Build history of the part. All positions in model axes, mm. Face numbers are marked on the shaded views. A direction names the side the tool comes from. Coordinates: 2 decimals unless noted, no trailing zeros. Write each loop counter-clockwise with the first axis right and the second up, starting at its lowest first coordinate (ties: lowest second). Pieces come first, ordered by that corner, then holes. Notation, with made-up numbers: (22, 68) -> (59, 68) arc R20 ccw to (59, 80) -> close; hole circle Ø5 at (-14.5, 89.5). An arc over 180 degrees is marked (long way). Write each question's results on one line, items separated by ' | '. Start each with the question number.
Q1. Drill centre lines: line 1 (Y direction, x = -17, z = -4.5); line 2 (Y direction, x = 2.5, z = -16.5); line 3 (X direction, y = 3.5, z = -12). Where is each one in solid material? Low to high.
Q2. Saw through at B-B on x = -17. Give the cut face in (y, z), and give its area (3 significant figures).
Q3. Saw through at C-C on z = -5. Give the cut face in (x, y), and give its area (3 significant figures).
Q4. Drop flat-ended pins along their axis: pin 1 Ø3.5 at (y, z) = (26.5, -26) entering from -X; pin 2 Ø9 at (x, y) = (17, 15) entering from +Z; pin 3 Ø1 at (x, y) = (-0.5, 14) entering from +Z; pin 4 Ø10 at (y, z) = (9, -25.5) entering from +X. Give the stop position or say it passes through.
Q5. Two-plate mould, pull along Z, no slides. Class the marked faces 1, 2, 3 and 4: released by +Z, released by -Z, zero draft, split by the parting line, or undercut.
Q6. Tool access for the marked faces 5, 6 and 7: list every direction of +Z, -Z, +X, -X, +Y, -Y with a clear straight run to the whole face (end or side of a thin tool).
Q7. Saw through at A-A on y = 15. Count the separate pieces of the cut face and the enclosed holes in it, and give its area (3 significant figures).
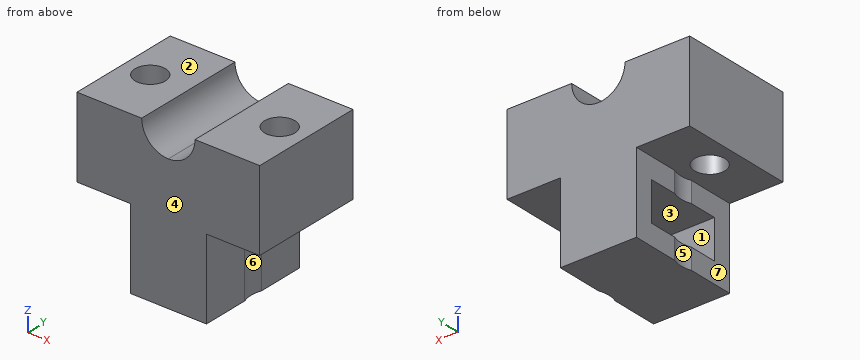
from build123d import *

# Parameters (mm, degrees)
SKETCH_1_W          = 48
SKETCH_1_H          = 20
EXTRUDE_1_DEPTH     = 30
SKETCH_2_W          = 14
SKETCH_2_H          = 30
CUT_EXTRUDE_1_DEPTH = 7
SKETCH_7_W          = 22
SKETCH_7_H          = 30
EXTRUDE_2_DEPTH     = 48
SKETCH_8_W          = 21
SKETCH_8_H          = 30
CUT_EXTRUDE_2_DEPTH = 14
SKETCH_9_W          = 21
SKETCH_9_H          = 30
CUT_EXTRUDE_3_DEPTH = 14
SKETCH_11_W         = 10.2
SKETCH_11_H         = 20.2
CUT_EXTRUDE_4_DEPTH = 56.497747702
SKETCH_13_R         = 4
CUT_EXTRUDE_5_DEPTH = 44.783558558
SKETCH_14_R         = 4
CUT_EXTRUDE_6_DEPTH = 44.783558558
FILLET_1_R          = 7
SKETCH1_W           = 10.2
SKETCH1_H           = 20.2
BOSS_EXTRUDE1_DEPTH = 4
SKETCH_20_R         = 7.5
CUT_EXTRUDE_8_DEPTH = 44.783558558


with BuildPart() as part:
    # Эскиз1 → Бобышка-Вытянуть1 (new body)
    with BuildSketch(Plane(origin=(0, 0, 0), x_dir=(1, 0, 0), z_dir=(0, 1, 0))):
        Rectangle(SKETCH_1_W, SKETCH_1_H)
    extrude(amount=EXTRUDE_1_DEPTH)

    # Эскиз2 → Вырез-Вытянуть1 (cut)
    with BuildSketch(Plane.XY.offset(10)):
        with Locations((0, 15)):
            Rectangle(SKETCH_2_W, SKETCH_2_H)
    extrude(amount=-CUT_EXTRUDE_1_DEPTH, mode=Mode.SUBTRACT)

    # Эскиз7 → Бобышка-Вытянуть2 (add)
    with BuildSketch(Plane(origin=(24, 0, 0), x_dir=(0, 0, -1), z_dir=(1, 0, 0))):
        with Locations((21, 15)):
            Rectangle(SKETCH_7_W, SKETCH_7_H)
    extrude(amount=-EXTRUDE_2_DEPTH)

    # Эскиз8 → Вырез-Вытянуть2 (cut)
    with BuildSketch(Plane(origin=(24, 0, 0), x_dir=(0, 0, -1), z_dir=(1, 0, 0))):
        with Locations((21.5, 15)):
            Rectangle(SKETCH_8_W, SKETCH_8_H)
    extrude(amount=-CUT_EXTRUDE_2_DEPTH, mode=Mode.SUBTRACT)

    # Эскиз9 → Вырез-Вытянуть3 (cut)
    with BuildSketch(Plane.ZY.offset(24)):
        with Locations((-21.5, 15)):
            Rectangle(SKETCH_9_W, SKETCH_9_H)
    extrude(amount=-CUT_EXTRUDE_3_DEPTH, mode=Mode.SUBTRACT)

    # Эскиз11 → Вырез-Вытянуть4 (cut, through all)
    with BuildSketch(Plane.ZY.offset(10)):
        with Locations((-21.5, 15)):
            Rectangle(SKETCH_11_W, SKETCH_11_H)
    extrude(amount=-CUT_EXTRUDE_4_DEPTH, mode=Mode.SUBTRACT)

    # Эскиз13 → Вырез-Вытянуть5 (cut, through all)
    with BuildSketch(Plane(origin=(0, 0, -11), x_dir=(-1, 0, 0), z_dir=(0, 0, -1))):
        with Locations((17, 15)):
            Circle(SKETCH_13_R)
    extrude(amount=-CUT_EXTRUDE_5_DEPTH, mode=Mode.SUBTRACT)

    # Эскиз14 → Вырез-Вытянуть6 (cut, through all)
    with BuildSketch(Plane(origin=(0, 0, -11), x_dir=(-1, 0, 0), z_dir=(0, 0, -1))):
        with Locations((-17, 15)):
            Circle(SKETCH_14_R)
    extrude(amount=-CUT_EXTRUDE_6_DEPTH, mode=Mode.SUBTRACT)

    # Скругление1
    fillet_1_edges = [part.edges().sort_by_distance(p)[0] for p in [
        (-7, 15, 3),
        (7, 15, 3),
    ]]
    fillet(fillet_1_edges, radius=FILLET_1_R - 0.0001)  # a hair under: the kernel refuses the full size

    # Sketch1 → Boss-Extrude1 (add)
    with BuildSketch(Plane(origin=(10, 0, 0), x_dir=(0, 0, -1), z_dir=(1, 0, 0))):
        with Locations((21.5, 15)):
            Rectangle(SKETCH1_W, SKETCH1_H)
    extrude(amount=-BOSS_EXTRUDE1_DEPTH)

    # Эскиз20 → Вырез-Вытянуть8 (cut, through all)
    with BuildSketch(Plane(origin=(0, 0, -11), x_dir=(-1, 0, 0), z_dir=(0, 0, -1))):
        with Locations((-17, 15)):
            Circle(SKETCH_20_R)
        with Locations((17, 15)):
            Circle(SKETCH_20_R)
    extrude(amount=CUT_EXTRUDE_8_DEPTH, mode=Mode.SUBTRACT)


solid = part.part
Returned:
1) line 1: y = 0 to 11, 19 to 30 | line 2: y = 0 to 4.9, 25.1 to 30 | line 3: x = -10 to 10
2) outline: (0, -11) -> (11, -11) -> (11, 10) -> (0, 10) -> close; (19, -11) -> (30, -11) -> (30, 10) -> (19, 10) -> close | area: 462 mm2
3) outline: (-24, 0) -> (24, 0) -> (24, 30) -> (-24, 30) -> close; hole circle Ø8 at (-17, 15); hole circle Ø8 at (17, 15) | area: 1,340 mm2
4) pin 1: stops at x = -10 | pin 2: stops at z = 10 | pin 3: stops at z = 3.07 | pin 4: stops at x = 10
5) face 1: undercut | face 2: released by +Z | face 3: undercut | face 4: zero draft
6) face 5: -Z, -X | face 6: -Z, +X | face 7: -Z, -X, +Y, -Y
7) separate pieces: 3 | enclosed holes: 0 | area: 836 mm2
